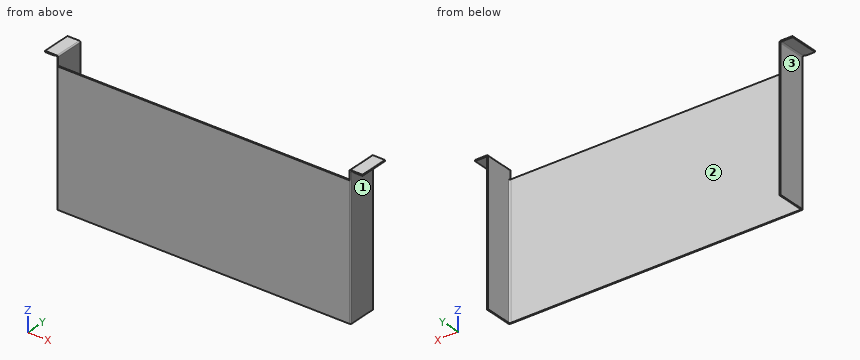
from build123d import *

# Parameters (mm, degrees)
BOSS_EXTRUDE1_DEPTH = 200
SKETCH2_W           = 1.75
SKETCH2_H           = 44.25
BOSS_EXTRUDE2_DEPTH = 15
SKETCH3_W           = 1.75
SKETCH3_H           = 44.25
BOSS_EXTRUDE3_DEPTH = 18
SKETCH4_W           = 1.75
SKETCH4_H           = 44.25
BOSS_EXTRUDE4_DEPTH = 18
FILLET1_R           = 1.75


with BuildPart() as part:
    # Sketch1 → Boss-Extrude1 (new body)
    with BuildSketch(Plane.XY):
        Polygon((-221.25, 0), (221.25, 0), (221.25, 42.5), (223, 42.5), (223, -1.75), (-223, -1.75), (-223, 42.5), (-221.25, 42.5), align=None)
    extrude(amount=BOSS_EXTRUDE1_DEPTH)

    # Sketch2 → Boss-Extrude2 (add)
    with BuildSketch(Plane.XY.offset(200)):
        with Locations((-222.125, 20.375)):
            Rectangle(SKETCH2_W, SKETCH2_H)
        with Locations((222.125, 20.375)):
            Rectangle(SKETCH2_W, SKETCH2_H)
    extrude(amount=BOSS_EXTRUDE2_DEPTH)

    # Sketch3 → Boss-Extrude3 (add)
    with BuildSketch(Plane(origin=(223, 0, 0), x_dir=(0, 0, -1), z_dir=(1, 0, 0))):
        with Locations((-214.125, 20.375)):
            Rectangle(SKETCH3_W, SKETCH3_H)
    extrude(amount=BOSS_EXTRUDE3_DEPTH)

    # Sketch4 → Boss-Extrude4 (add)
    with BuildSketch(Plane.ZY.offset(223)):
        with Locations((214.125, 20.375)):
            Rectangle(SKETCH4_W, SKETCH4_H)
    extrude(amount=BOSS_EXTRUDE4_DEPTH)

    # Fillet1
    # the kernel refuses this fillet: 1.75 mm, written as the material it adds along each edge
    with BuildSketch(Plane(origin=(-221.25, 0, 0), x_dir=(1, 0, 0), z_dir=(0, 0, 1))) as fillet1_piece_1:
        with BuildLine():
            CenterArc((FILLET1_R, FILLET1_R), FILLET1_R, 180, 90)
            Line((0, FILLET1_R), (0, 0))
            Line((0, 0), (FILLET1_R, 0))
        make_face()
    extrude(amount=200)
    with BuildSketch(Plane(origin=(221.25, 0, 0), x_dir=(-1, 0, 0), z_dir=(0, 0, 1))) as fillet1_piece_2:
        with BuildLine():
            CenterArc((FILLET1_R, -FILLET1_R), FILLET1_R, 90, 90)
            Line((0, -FILLET1_R), (0, 0))
            Line((0, 0), (FILLET1_R, 0))
        make_face()
    extrude(amount=200)
    with BuildSketch(Plane(origin=(223, -1.75, 213.25), x_dir=(1, 0, 0), z_dir=(0, 1, 0)), Plane(origin=(-223, -1.75, 213.25), x_dir=(0, 0, -1), z_dir=(0, 1, 0))) as fillet1_piece_3:
        with BuildLine():
            CenterArc((FILLET1_R, FILLET1_R), FILLET1_R, 180, 90)
            Line((0, FILLET1_R), (0, 0))
            Line((0, 0), (FILLET1_R, 0))
        make_face()
    extrude(amount=44.25)
    # the kernel refuses this fillet: 1.75 mm, written as the material it takes off along each edge
    with BuildSketch(Plane(origin=(-221.25, -6.125, 215), x_dir=(0, 0, -1), z_dir=(0, 1, 0))) as fillet1_2_piece_1:
        with BuildLine():
            CenterArc((FILLET1_R, FILLET1_R), FILLET1_R, 180, 90)
            Line((0, FILLET1_R), (0, 0))
            Line((0, 0), (FILLET1_R, 0))
        make_face()
    extrude(amount=53, mode=Mode.SUBTRACT)
    with BuildSketch(Plane(origin=(221.25, -6.125, 215), x_dir=(0, 0, -1), z_dir=(0, 1, 0))) as fillet1_2_piece_2:
        with BuildLine():
            CenterArc((FILLET1_R, -FILLET1_R), FILLET1_R, 90, 90)
            Line((0, -FILLET1_R), (0, 0))
            Line((0, 0), (FILLET1_R, 0))
        make_face()
    extrude(amount=53, mode=Mode.SUBTRACT)
    with BuildSketch(Plane(origin=(223, -1.75, 211.5), x_dir=(-1, 0, 0), z_dir=(0, 0, -1))) as fillet1_2_piece_3:
        with BuildLine():
            CenterArc((FILLET1_R, FILLET1_R), FILLET1_R, 180, 90)
            Line((0, FILLET1_R), (0, 0))
            Line((0, 0), (FILLET1_R, 0))
        make_face()
    extrude(amount=215.875, mode=Mode.SUBTRACT)
    with BuildSketch(Plane(origin=(-223, -1.75, 211.5), x_dir=(1, 0, 0), z_dir=(0, 0, -1))) as fillet1_2_piece_4:
        with BuildLine():
            CenterArc((FILLET1_R, -FILLET1_R), FILLET1_R, 90, 90)
            Line((0, -FILLET1_R), (0, 0))
            Line((0, 0), (FILLET1_R, 0))
        make_face()
    extrude(amount=215.875, mode=Mode.SUBTRACT)
    with BuildSketch(Plane(origin=(-224.75, -1.75, 211.5), x_dir=(1, 0, 0), z_dir=(0, 0, -1))) as fillet1_2_piece_5:
        with BuildLine():
            CenterArc((1.75 + FILLET1_R, -FILLET1_R), FILLET1_R, 90, 90)
            Line((1.75, -FILLET1_R), (1.75, 0))
            Line((1.75, 0), (1.75 + FILLET1_R, 0))
        make_face()
    revolve(axis=Axis((-224.75, -1.75, 211.5), (0, -1, 0)), revolution_arc=233.296989237, mode=Mode.SUBTRACT)
    with BuildSketch(Plane(origin=(224.75, -1.75, 211.5), x_dir=(0.5976672776328118, 0, -0.80174423929766), z_dir=(-0.80174423929766, 0, -0.5976672776328118))) as fillet1_2_piece_6:
        with BuildLine():
            CenterArc((1.75 + FILLET1_R, -FILLET1_R), FILLET1_R, 90, 90)
            Line((1.75, -FILLET1_R), (1.75, 0))
            Line((1.75, 0), (1.75 + FILLET1_R, 0))
        make_face()
    revolve(axis=Axis((224.75, -1.75, 211.5), (0, -1, 0)), revolution_arc=233.296989237, mode=Mode.SUBTRACT)


solid = part.part
Work out the finished part from the listing and answer in its coordinate system (mm). Face numbers are marked on the shaded views. A direction names the side the tool comes from. Coordinates: 2 decimals unless noted, no trailing zeros. Write each loop counter-clockwise with the first axis right and the second up, starting at its lowest first coordinate (ties: lowest second). Pieces come first, ordered by that corner, then holes. Notation, with made-up numbers: M 81,-17 L 94,-17 A21 ccw 94,5 Z; hole C -18.75,13 d5. An arc over 180 degrees is marked long. Use one line per item in the form item = value. Start each with the question number.
1. The part is cut by section C-C (x = -79). Give the vertices of the cut face in (y, z), plus the area to 3 significant figures.
2. Straight lines are drawn through the part: probe 1 along X at (y, z) = (35, 114.5); probe 2 along Y at (x, z) = (-204, 161). For each, find the intervals that lie inside material, in ascending order. Write a range as from..to.
3. The part is cut by section B-B (z = 35). Give the vertices of the cut face in (x, y), plus the area to 3 significant figures.
4. Each of these flat-tipped pins is pushed along its axis until it touches: P1, Ø21, axis at y = 28.5, z = 75, coming from the -X side; P2, Ø1.8, axis at x = 80, y = -0.5, coming from the +Z side; P3, Ø8, axis at x = 85, z = 38.5, coming from the +Y side. Where does it stop, or does it pass through?
5. A tool of negligible diameter and unlimited length cuts with its end or side. For the marked faces 1, 2 and 3, from which of +Z, -Z, +X, -X, +Y, -Y can it reach the whole face along a straight path? Write none if from no direction.
6. The part is cut by section A-A (y = 12). Give the vertices of the cut face in (x, z), plus the area to 4 significant figures.
Evaluation:
q1.outline = M -1.75,0 L 0,0 L 0,200 L -1.75,200 Z
q1.area = 350 mm^2
q2.probe_1 = -223..-221.25, 221.25..223
q2.probe_2 = -1.75..0
q3.outline = M -223,0 A1.75 ccw -221.25,-1.75 L 221.25,-1.75 A1.75 ccw 223,0 L 223,42.5 L 221.25,42.5 L 221.25,1.75 A1.75 cw 219.5,0 L -219.5,0 A1.75 cw -221.25,1.75 L -221.25,42.5 L -223,42.5 Z
q3.area = 929 mm^2
q4.P1 = -223
q4.P2 = 200
q4.P3 = 0
q5.face_1 = -Z, +X, +Y, -Y
q5.face_2 = +Z, -Z, +Y
q5.face_3 = -Z, -X, +Y, -Y
q6.outline = M -241,213.25 L -224.75,213.25 A1.75 cw -223,211.5 L -223,0 L -221.25,0 L -221.25,213.25 A1.75 ccw -223,215 L -241,215 Z; M 221.25,0 L 223,0 L 223,211.5 A1.75 cw 224.75,213.25 L 241,213.25 L 241,215 L 223,215 A1.75 ccw 221.25,213.25 Z
q6.area = 815.5 mm^2
